Can you work these out from the model? Positions are in its coordinate system, mm. A direction names the side the tool comes from. Coordinates: 2 decimals unless noted, no trailing zeros. Loops run counter-clockwise (first coordinate to the right, second up) from the corner with the lowest first, then second, coordinate; pieces in that order, holes last.
```python
from build123d import *

# Parameters (mm, degrees)
AUFSATZ_LINEAR_AUSTRAGEN1_DEPTH      = 25
AUFSATZ_LINEAR_AUSTRAGEN1_DEPTH_BACK = 25
SKIZZE1_R                            = 13
SKIZZE2_R                            = 13
AUFSATZ_LINEAR_AUSTRAGEN2_DEPTH      = 150
SKIZZE4_R                            = 5
AUFSATZ_LINEAR_AUSTRAGEN3_DEPTH      = 16
SKIZZE5_R                            = 12.5
AUFSATZ_LINEAR_AUSTRAGEN4_DEPTH      = 8
SKIZZE6_R                            = 5
AUFSATZ_LINEAR_AUSTRAGEN5_DEPTH      = 1
SCHNITT_LINEAR_AUSTRAGEN2_REACH      = 183.204
SKIZZE7_R                            = 1.25
SCHNITT_LINEAR_AUSTRAGEN3_REACH      = 171.901
SCHNITT_LINEAR_AUSTRAGEN3_END_RADIUS = 13
SKIZZE8_W                            = 15
SKIZZE8_H                            = 25


with BuildPart() as part:
    # Skizze1 → Aufsatz-Linear austragen1 (new, two sides: drawn at the far end of the back side and taken through both)
    with BuildSketch(Plane(origin=(0, 0, 0), x_dir=(0, 0, -1), z_dir=(1, 0, 0)).offset(-AUFSATZ_LINEAR_AUSTRAGEN1_DEPTH_BACK)):
        Circle(SKIZZE1_R)
    extrude(amount=AUFSATZ_LINEAR_AUSTRAGEN1_DEPTH + AUFSATZ_LINEAR_AUSTRAGEN1_DEPTH_BACK)

    # Skizze2 → Aufsatz-Linear austragen2 (add)
    with BuildSketch(Plane.XY):
        with Locations(Location((0, 0, 0), (0, 0, 90))):
            Circle(SKIZZE2_R)
    extrude(amount=AUFSATZ_LINEAR_AUSTRAGEN2_DEPTH)

    # Skizze4 → Aufsatz-Linear austragen3 (add)
    with BuildSketch(Plane.XY.offset(150)):
        Circle(SKIZZE4_R)
    extrude(amount=AUFSATZ_LINEAR_AUSTRAGEN3_DEPTH)

    # Skizze5 → Aufsatz-Linear austragen4 (add)
    with BuildSketch(Plane.XY.offset(166)):
        Circle(SKIZZE5_R)
    extrude(amount=-AUFSATZ_LINEAR_AUSTRAGEN4_DEPTH)

    # Skizze6 → Aufsatz-Linear austragen5 (add)
    with BuildSketch(Plane.XY.offset(166)):
        Circle(SKIZZE6_R)
    extrude(amount=AUFSATZ_LINEAR_AUSTRAGEN5_DEPTH)

    # Skizze7 → Schnitt-Linear austragen2 (cut, up to next)
    with BuildSketch(Plane.XY.offset(166), mode=Mode.PRIVATE) as schnitt_linear_austragen2_sk1:
        with Locations((-11, 0)):
            Circle(SKIZZE7_R)
    schnitt_linear_austragen2_tool1 = extrude(schnitt_linear_austragen2_sk1.sketch, amount=-SCHNITT_LINEAR_AUSTRAGEN2_REACH, mode=Mode.PRIVATE) & part.part
    # Skizze7 → Schnitt-Linear austragen2 (cut, up to next)
    with BuildSketch(Plane.XY.offset(166), mode=Mode.PRIVATE) as schnitt_linear_austragen2_sk2:
        with Locations((-7.778174593, 7.778174593)):
            Circle(SKIZZE7_R)
    schnitt_linear_austragen2_tool2 = extrude(schnitt_linear_austragen2_sk2.sketch, amount=-SCHNITT_LINEAR_AUSTRAGEN2_REACH, mode=Mode.PRIVATE) & part.part
    # Skizze7 → Schnitt-Linear austragen2 (cut, up to next)
    with BuildSketch(Plane.XY.offset(166), mode=Mode.PRIVATE) as schnitt_linear_austragen2_sk3:
        with Locations((7.778174593, 7.778174593)):
            Circle(SKIZZE7_R)
    schnitt_linear_austragen2_tool3 = extrude(schnitt_linear_austragen2_sk3.sketch, amount=-SCHNITT_LINEAR_AUSTRAGEN2_REACH, mode=Mode.PRIVATE) & part.part
    # Skizze7 → Schnitt-Linear austragen2 (cut, up to next)
    with BuildSketch(Plane.XY.offset(166), mode=Mode.PRIVATE) as schnitt_linear_austragen2_sk4:
        with Locations((11, 0)):
            Circle(SKIZZE7_R)
    schnitt_linear_austragen2_tool4 = extrude(schnitt_linear_austragen2_sk4.sketch, amount=-SCHNITT_LINEAR_AUSTRAGEN2_REACH, mode=Mode.PRIVATE) & part.part
    # Skizze7 → Schnitt-Linear austragen2 (cut, up to next)
    with BuildSketch(Plane.XY.offset(166), mode=Mode.PRIVATE) as schnitt_linear_austragen2_sk5:
        with Locations((7.778174593, -7.778174593)):
            Circle(SKIZZE7_R)
    schnitt_linear_austragen2_tool5 = extrude(schnitt_linear_austragen2_sk5.sketch, amount=-SCHNITT_LINEAR_AUSTRAGEN2_REACH, mode=Mode.PRIVATE) & part.part
    # Skizze7 → Schnitt-Linear austragen2 (cut, up to next)
    with BuildSketch(Plane.XY.offset(166), mode=Mode.PRIVATE) as schnitt_linear_austragen2_sk6:
        with Locations((-7.778174593, -7.778174593)):
            Circle(SKIZZE7_R)
    schnitt_linear_austragen2_tool6 = extrude(schnitt_linear_austragen2_sk6.sketch, amount=-SCHNITT_LINEAR_AUSTRAGEN2_REACH, mode=Mode.PRIVATE) & part.part
    # Skizze7 → Schnitt-Linear austragen2 (cut, up to next)
    with BuildSketch(Plane.XY.offset(166), mode=Mode.PRIVATE) as schnitt_linear_austragen2_sk7:
        with Locations((0, -11)):
            Circle(SKIZZE7_R)
    schnitt_linear_austragen2_tool7 = extrude(schnitt_linear_austragen2_sk7.sketch, amount=-SCHNITT_LINEAR_AUSTRAGEN2_REACH, mode=Mode.PRIVATE) & part.part
    # Skizze7 → Schnitt-Linear austragen2 (cut, up to next)
    with BuildSketch(Plane.XY.offset(166), mode=Mode.PRIVATE) as schnitt_linear_austragen2_sk8:
        with Locations((0, 11)):
            Circle(SKIZZE7_R)
    schnitt_linear_austragen2_tool8 = extrude(schnitt_linear_austragen2_sk8.sketch, amount=-SCHNITT_LINEAR_AUSTRAGEN2_REACH, mode=Mode.PRIVATE) & part.part
    add(schnitt_linear_austragen2_tool1.solids().sort_by_distance((-11, 0, 166))[0], mode=Mode.SUBTRACT)
    add(schnitt_linear_austragen2_tool2.solids().sort_by_distance((-7.778175, 7.778175, 166))[0], mode=Mode.SUBTRACT)
    add(schnitt_linear_austragen2_tool3.solids().sort_by_distance((7.778175, 7.778175, 166))[0], mode=Mode.SUBTRACT)
    add(schnitt_linear_austragen2_tool4.solids().sort_by_distance((11, 0, 166))[0], mode=Mode.SUBTRACT)
    add(schnitt_linear_austragen2_tool5.solids().sort_by_distance((7.778175, -7.778175, 166))[0], mode=Mode.SUBTRACT)
    add(schnitt_linear_austragen2_tool6.solids().sort_by_distance((-7.778175, -7.778175, 166))[0], mode=Mode.SUBTRACT)
    add(schnitt_linear_austragen2_tool7.solids().sort_by_distance((0, -11, 166))[0], mode=Mode.SUBTRACT)
    add(schnitt_linear_austragen2_tool8.solids().sort_by_distance((0, 11, 166))[0], mode=Mode.SUBTRACT)

    # Schnitt-Linear austragen3: up to this cylinder (the profile starts inside it)
    schnitt_linear_austragen3_end = Plane(origin=(0, 0, 72.5), z_dir=(0, 0, -1)) * Cylinder(SCHNITT_LINEAR_AUSTRAGEN3_END_RADIUS, 370.802, mode=Mode.PRIVATE)
    # Skizze8 → Schnitt-Linear austragen3 (cut, up to the surface)
    with BuildSketch(Plane(origin=(0, 5.771219274, 0), x_dir=(1, 0, 0), z_dir=(0, 1, 0)), mode=Mode.PRIVATE) as schnitt_linear_austragen3_sk1:
        with Locations((0, -72.5)):
            Rectangle(SKIZZE8_W, SKIZZE8_H)
    schnitt_linear_austragen3_tool1 = extrude(schnitt_linear_austragen3_sk1.sketch, amount=SCHNITT_LINEAR_AUSTRAGEN3_REACH, mode=Mode.PRIVATE) & schnitt_linear_austragen3_end
    add(schnitt_linear_austragen3_tool1.solids().sort_by_distance((0, 5.771219, 72.5))[0], mode=Mode.SUBTRACT)


solid = part.part
```
(1) If I drill on probe 1 along Z at (x, y) = (3.5, 7); probe 2 along Z at (x, y) = (-4, 10.5); probe 3 along Y at (x, z) = (11, 161.25), over which ranges is the centre line in solid material (lowest first)?
Check values:
probe 1: z = -10.95 to 60, 85 to 150, 158 to 166
probe 2: z = -7.66 to 60, 85 to 150, 158 to 166
probe 3: y = -5.94 to -1.25, 1.25 to 5.94
(2) I want a section at B-B on z = 18.5. Write out the boundary of the cut face in (x, y).
Check values:
outline: circle Ø26 at (0, 0)
(3) Which directions (+Z, -Z, +X, -X, +Y, -Y) give clear straight access to the entire face, cutting with the end or side of a thin tool? Please do faces 4 (the cylindrical face through (-1.08, -4.88, 153.94)), 5 (the flat face through (-25, 0, 0)), 6 (the flat face through (25, 0, 0)), 7 (the cylindrical face through (-1.08, -4.88, 166.49)), 8 (the flat face through (7.5, 8, 73)).
Check values:
face 4: none
face 5: +Z, -Z, -X, +Y, -Y
face 6: +Z, -Z, +X, +Y, -Y
face 7: +Z
face 8: +Y
(4) If we mould it in two halves opening along X, with no side actions, what happens to faces 1 (the flat face through (0, 9, 85)), 2 (the flat face through (0, 0, 167)), 3 (the cylindrical face through (11.923, 3.755, 162.056))? For each: released by +X, released by -X, zero draft, split by the parting line, or undercut.
Check values:
face 1: undercut
face 2: zero draft
face 3: split by the parting line
(5) I want a section at A-A on z = 67.5. Write out the boundary of the cut face in (x, y), then the cut area to 3 significant figures.
Check values:
outline: (-7.5, 5.77) - (-7.5, 10.62) arc R13 ccw (long way) to (7.5, 10.62) - (7.5, 5.77) - close
area: 434 mm2
(6) I'm going to push flat-ended pins straight in: pin 1 (4.5 mm diameter, centred on x = -2, z = 69.5, fed in from +Y); pin 2 (12 mm diameter, centred on x = 9.5, z = 35.5, fed in from +Y); pin 3 (2 mm diameter, centred on x = 7.78, y = -7.78, fed in from -Z); pin 4 (2 mm diameter, centred on x = 1, z = 32.5, fed in from +Y). Where does each tip first touch, or does it pass through?
Check values:
pin 1: stops at y = 5.77
pin 2: stops at y = 12.52
pin 3: stops at z = -11.09
pin 4: stops at y = 13
